The model under review builds one solid part; all positions refer to its coordinate system, in mm. A direction names the side the tool comes from. Coordinates: 2 decimals unless noted, no trailing zeros. Write each loop counter-clockwise with the first axis right and the second up, starting at its lowest first coordinate (ties: lowest second). Pieces come first, ordered by that corner, then holes. Notation, with made-up numbers: M 32,5 L 75,5 A23 cw 75,30 Z; hole C 51.25,80 d8. An arc over 180 degrees is marked long. Answer as a JSON object with one key per item and string values.
```python
from build123d import *

# Parameters (mm, degrees)
F0_R     = 20
F1_DEPTH = 171.5
F2_R     = 12.5
F3_DEPTH = 28.52
F4_R     = 12.5
F5_DEPTH = 28.52
F6_R     = 10
F7_DEPTH = 25
F8_R     = 10
F9_DEPTH = 25


with BuildPart() as f1:
    # F0 (on Right) → F1 (new body)
    with BuildSketch(Plane.YZ):
        Circle(F0_R)
    extrude(amount=F1_DEPTH)

    # F2 (on face) → F3 (join)
    with BuildSketch(Plane(origin=(0, 0, 0), x_dir=(0, -1, 0), z_dir=(-1, 0, 0))):
        Circle(F2_R)
    extrude(amount=F3_DEPTH)

    # F4 (on face) → F5 (join)
    with BuildSketch(Plane.YZ.offset(171.5)):
        Circle(F4_R)
    extrude(amount=F5_DEPTH)

    # F6 (on face) → F7 (join)
    with BuildSketch(Plane(origin=(-28.52, 0, 0), x_dir=(0, -1, 0), z_dir=(-1, 0, 0))):
        Circle(F6_R)
    extrude(amount=F7_DEPTH)

    # F8 (on face) → F9 (join)
    with BuildSketch(Plane.YZ.offset(200.02)):
        Circle(F8_R)
    extrude(amount=F9_DEPTH)


solid = f1.part
```
(1) Add section C-C on x = -10. Give the boundary of the cut face in (y, z), and give its area (3 significant figures).
Results list:
{"outline": "C 0,0 d25", "area": "491 mm²"}
(2) Wall thickness on line 1 along X through (y, z) = (12.5, 6.5); line 2 along Z through (x, y) = (60, 0); line 3 along Z through (x, y) = (-11.5, -7.5): over which ranges is each line inside the solid? List them lowest first. Write a range as from..to.
Results list:
{"line 1": "0..171.5", "line 2": "-20..20", "line 3": "-10..10"}
(3) Add section D-D on z = -16. Give the boundary of the cut face in (x, y), and give its area (3 significant figures).
Results list:
{"outline": "M 0,-12 L 171.5,-12 L 171.5,12 L 0,12 Z", "area": "4,120 mm²"}
(4) Add section A-A on z = 0. Give the boundary of the cut face in (x, y), and give its area (3 significant figures).
Results list:
{"outline": "M -53.52,-10 L -28.52,-10 L -28.52,-12.5 L 0,-12.5 L 0,-20 L 171.5,-20 L 171.5,-12.5 L 200.02,-12.5 L 200.02,-10 L 225.02,-10 L 225.02,10 L 200.02,10 L 200.02,12.5 L 171.5,12.5 L 171.5,20 L 0,20 L 0,12.5 L -28.52,12.5 L -28.52,10 L -53.52,10 Z", "area": "9,290 mm²"}
(5) For pin 1 Ø3 at (x, y) = (92.5, 5) entering from +Z; pin 2 Ø12 at (x, y) = (146.5, 3.5) entering from +Z; pin 3 Ø3 at (y, z) = (-5.5, -13) entering from -X, all flat-tipped, find the tip position at first contact; note any pin that passes through.
Results list:
{"pin 1": "z = 19.69", "pin 2": "z = 20", "pin 3": "x = 0"}
(6) For faces 1 (the face through (200.02, -0.1, 10.2)), 2 (the face through (84.55, -4.336, -19.524)), 3 (the face through (-40.84, 2.17, -9.76)), list the 3-axis set-ups (+Z, -Z, +X, -X, +Y, -Y) from which the entire face can be reached by the end or side of a thin tool; tool diameter is ignored.
Results list:
{"face 1": "+X", "face 2": "+X, -X", "face 3": "-X"}
